Check sheet for the modelled part. Datum: model origin and axes. Units: mm. Face numbers are marked on the shaded views. A direction names the side the tool comes from. Give positions to 0.01 mm unless a question says otherwise; leave off trailing zeros. Order: outer loops, then holes, each group sorted by start corner. A loop starts at its lowest first (then second) coordinate and runs counter-clockwise, first axis right, second up.
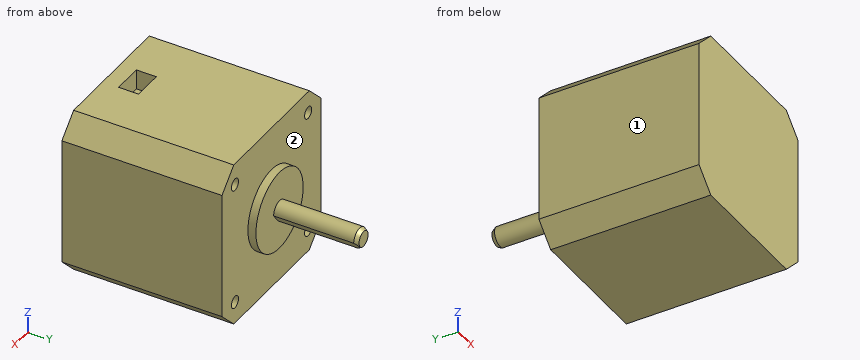
from build123d import *

# Parameters (mm, degrees)
SKETCH1_W                 = 42
SKETCH1_H                 = 42
BOSS_EXTRUDE1_DEPTH       = 40
F_3_0MM_DOWEL_HOLE1_D     = 3
F_3_0MM_DOWEL_HOLE1_DEPTH = 4.5
F_3_0MM_DOWEL_HOLE1_TIP   = 0.901290929
SKETCH2_R                 = 10
BOSS_EXTRUDE2_DEPTH       = 2
BOSS_EXTRUDE3_DEPTH       = 23
SKETCH10_W                = 7.5
SKETCH10_H                = 5
CUT_EXTRUDE1_DEPTH        = 5
CHAMFER2_SIZE             = 5


with BuildPart() as part:
    # Sketch1 → Boss-Extrude1 (new body)
    with BuildSketch(Plane(origin=(0, 0, 0), x_dir=(1, 0, 0), z_dir=(0, 1, 0))):
        Rectangle(SKETCH1_W, SKETCH1_H)
    extrude(amount=BOSS_EXTRUDE1_DEPTH)

    # Ø3.0mm Dowel Hole1
    with Locations(Plane(origin=(0, 40, 0), x_dir=(1, 0, 0), z_dir=(0, 1, 0))):
        with Locations((-15.5, 15.5), (15.5, 15.5), (15.5, -15.5), (-15.5, -15.5)):
            Hole(F_3_0MM_DOWEL_HOLE1_D / 2, depth=F_3_0MM_DOWEL_HOLE1_DEPTH)
            with Locations((0, 0, -(F_3_0MM_DOWEL_HOLE1_DEPTH + F_3_0MM_DOWEL_HOLE1_TIP / 2))):  # 118° drill point
                Cone(0, F_3_0MM_DOWEL_HOLE1_D / 2, F_3_0MM_DOWEL_HOLE1_TIP, mode=Mode.SUBTRACT)

    # Sketch2 → Boss-Extrude2 (add)
    with BuildSketch(Plane(origin=(0, 40, 0), x_dir=(1, 0, 0), z_dir=(0, 1, 0))):
        with Locations(Location((0, 0, 0), (0, 0, 90))):
            Circle(SKETCH2_R)
    extrude(amount=BOSS_EXTRUDE2_DEPTH)

    # Sketch4 → Boss-Extrude3 (add)
    with BuildSketch(Plane(origin=(0, 40, 0), x_dir=(1, 0, 0), z_dir=(0, 1, 0))):
        with BuildLine():
            Line((0.7, 2.4), (2.5, 0))
            ThreePointArc((2.5, 0), (-2, -1.5), (0.7, 2.4))
        make_face()
    extrude(amount=BOSS_EXTRUDE3_DEPTH)

    # Sketch10 → Cut-Extrude1 (cut)
    with BuildSketch(Plane.XY.offset(21)):
        with Locations((0, 6.5)):
            Rectangle(SKETCH10_W, SKETCH10_H)
    extrude(amount=-CUT_EXTRUDE1_DEPTH, mode=Mode.SUBTRACT)

    # Chamfer1: read off the stored shape, not the designer's step
    # Chamfer1 outline → Chamfer1 (revolve, cut)
    with BuildSketch(Plane.XY):
        Polygon((2.5, 63), (1.922649731, 63), (2.5, 62), align=None)
    revolve(axis=Axis((0, 0, 0), (0, 1, 0)), mode=Mode.SUBTRACT)

    # Chamfer2
    chamfer2_edges = [part.edges().sort_by_distance(p)[0] for p in [
        (21, 20, 21),
        (-21, 20, 21),
        (-21, 20, -21),
        (21, 20, -21),
    ]]
    chamfer(chamfer2_edges, length=CHAMFER2_SIZE)


solid = part.part
1) Section check C-C, the plane z = 11. Record the cut outline in (x, y).
Recorded:
outline: (-21, 0) - (21, 0) - (21, 40) - (-21, 40) - close
2) Section check B-B, the plane y = 18. Record the cut outline in (x, z), then the cut area to 3 significant figures.
Recorded:
outline: (-21, -16) - (-16, -21) - (16, -21) - (21, -16) - (21, 16) - (16, 21) - (-16, 21) - (-21, 16) - close
area: 1,710 mm2
3) Depth check by flat-ended pin: pin 1 Ø1.5 at (y, z) = (7.5, 18) entering from +X; pin 2 Ø3.5 at (x, z) = (15.5, 15.5) entering from +Y; pin 3 Ø6 at (y, z) = (45.5, 12.5) entering from +X. Enter the tip coordinate at first touch or a pass-through.
Recorded:
pin 1: stops at x = 19.75
pin 2: stops at y = 40
pin 3: passes through
4) Section check D-D, the plane z = -4. Record the cut outline in (x, y).
Recorded:
outline: (-21, 0) - (21, 0) - (21, 40) - (9.17, 40) - (9.17, 42) - (-9.17, 42) - (-9.17, 40) - (-21, 40) - close
5) Set-up check for the marked faces 1 and 2: record each of +Z, -Z, +X, -X, +Y, -Y from which the full face is reachable in a straight line by a thin tool's end or side.
Recorded:
face 1: +Z, -Z, -X, +Y, -Y
face 2: +Y
6) Section check A-A, the plane x = 0. Record the cut outline in (y, z), then the cut area to 3 significant figures.
Recorded:
outline: (0, -21) - (40, -21) - (40, -10) - (42, -10) - (42, -2.5) - (62, -2.5) - (63, -1.92) - (63, 1.92) - (62, 2.5) - (42, 2.5) - (42, 10) - (40, 10) - (40, 21) - (9, 21) - (9, 16) - (4, 16) - (4, 21) - (0, 21) - close
area: 1,800 mm2
7) Material ranges on L1, parallel to Z at x = 15.5, y = 37.8; L2, parallel to Z at x = -15, y = 37, recorded low to high.
Recorded:
L1: z = -21 to -17, -14 to 14, 17 to 21
L2: z = -21 to -16.91, -14.09 to 14.09, 16.91 to 21
